from build123d import *

# Parameters (mm, degrees)
SKETCH037_W      = 2
SKETCH037_H      = 37
EXTRUDE036_DEPTH = 1
FILLET012_R      = 0.25
SKETCH038_W      = 13.25
SKETCH038_H      = 36
EXTRUDE037_DEPTH = 2
SKETCH031_W      = 37
SKETCH031_H      = 2.5
EXTRUDE029_DEPTH = 120
SKETCH030_W      = 56
SKETCH030_H      = 13.5
EXTRUDE028_DEPTH = 41
SKETCH036_W      = 120
SKETCH036_H      = 8
EXTRUDE035_DEPTH = 2
FILLET011_R      = 1
FILLET013_R      = 4
FILLET014_R      = 1


with BuildPart() as velcrobands:
    # Sketch037 → Extrude036 (new body)
    with BuildSketch(Plane.XY.offset(5.5)):
        with Locations((174, 26.5)):
            Rectangle(SKETCH037_W, SKETCH037_H)
        with Locations((147, 26.5)):
            Rectangle(SKETCH037_W, SKETCH037_H)
    extrude(amount=EXTRUDE036_DEPTH)

    # Fillet012
    fillet012_edges = [velcrobands.edges().sort_by_distance(p)[0] for p in [
        (148, 26.5, 6.5),
        (146, 26.5, 6.5),
        (173, 26.5, 6.5),
        (175, 26.5, 6.5),
    ]]
    fillet(fillet012_edges, radius=FILLET012_R)


with BuildPart() as sensorcuts:
    # Sketch038 → Extrude037 (new body)
    with BuildSketch(Plane.XY.offset(-0.75)):
        with Locations((151.375, 26.5)):
            Rectangle(SKETCH038_W, SKETCH038_H)
    extrude(amount=-EXTRUDE037_DEPTH)


with BuildPart() as extrude029:
    # Sketch031 → Extrude029 (new body)
    with BuildSketch(Plane.YZ.offset(56)):
        with Locations((26.412533, 0.5)):
            Rectangle(SKETCH031_W, SKETCH031_H)
    extrude(amount=EXTRUDE029_DEPTH)


with BuildPart() as band002:
    # Sketch030 → Extrude028 (new body)
    with BuildSketch(Plane.XZ.offset(-6)):
        Polygon((175, 5.5), (60, 5.5), (60, 17.5), (-4, 17.5), (-4, 2.5), (-122, 2.5), (-122, -2.5), (175, -2.5), align=None)
        with Locations((28, 6.75)):
            Rectangle(SKETCH030_W, SKETCH030_H, mode=Mode.SUBTRACT)
    extrude(amount=-EXTRUDE028_DEPTH)

    # Cut002: cut Extrude029
    add(extrude029.part, mode=Mode.SUBTRACT)

    # Cut005: cut sensorCuts
    add(sensorcuts.part, mode=Mode.SUBTRACT)


with BuildPart() as fillet014:
    # Sketch036 → Extrude035 (new body)
    with BuildSketch(Plane.XY.offset(2.5)):
        with Locations((-62, 43)):
            Rectangle(SKETCH036_W, SKETCH036_H)
        with Locations((-62, 10)):
            Rectangle(SKETCH036_W, SKETCH036_H)
    extrude(amount=EXTRUDE035_DEPTH)

    # Fillet011
    fillet011_edges = [fillet014.edges().sort_by_distance(p)[0] for p in [
        (-62, 14, 4.5),
        (-62, 6, 4.5),
        (-62, 47, 4.5),
        (-62, 39, 4.5),
    ]]
    fillet(fillet011_edges, radius=FILLET011_R)

    # Fusion011: union velcroBands, band002
    add(velcrobands.part)
    add(band002.part)

    # Fillet013
    fillet013_edges = [fillet014.edges().sort_by_distance(p)[0] for p in [
        (60, 26.5, 5.5),
        (60, 26.5, 17.5),
        (-4, 26.5, 17.5),
        (0, 26.5, 0),
        (0, 26.5, 13.5),
        (56, 26.5, 13.5),
    ]]
    fillet(fillet013_edges, radius=FILLET013_R)

    # Fillet014
    fillet014_edges = [fillet014.edges().sort_by_distance(p)[0] for p in [
        (119.5, 6, 5.5),
        (26.5, 6, -2.5),
        (28, 6, 17.5),
        (28, 6, 13.5),
        (119.5, 47, 5.5),
        (26.5, 47, -2.5),
        (158, 26.5, -2.5),
        (151.375, 8.5, -2.5),
        (144.75, 26.5, -2.5),
        (151.375, 44.5, -2.5),
        (28, 47, 17.5),
        (56, 6.956266, 0),
        (56, 45.956266, 0),
        (28, 47, 13.5),
        (56, 26.412533, 1.75),
        (158, 8.5, -1.625),
        (158, 44.5, -1.625),
        (144.75, 8.5, -1.625),
        (144.75, 44.5, -1.625),
    ]]
    fillet(fillet014_edges, radius=FILLET014_R)


solid = fillet014.part
Geometry: final body of the model. Coordinates: model frame, mm. A direction names the side the tool comes from. Give positions to 0.01 mm unless a question says otherwise; leave off trailing zeros. Order: outer loops, then holes, each group sorted by start corner. A loop starts at its lowest first (then second) coordinate and runs counter-clockwise, first axis right, second up. Notation, with made-up numbers: (79, -20) - (136, -20) arc R19 cw to (136, 10) - close; hole circle Ø10 at (-1, -8.75). An arc over 180 degrees is marked (long way). Use CSV: the item, a comma, the result in double quotes.
1. Access query for faces 1 (the face through (115, 26, -0.75)), 2 (the face through (-64, 43, 4.5)), 3 (the face through (28, 26, 13.5)). Directions: +Z, -Z, +X, -X, +Y, -Y. A direction counts if a zero-diameter tool reaches every point of the face in a straight line with its end or side. Return the directions, or none.
Answers below:
face 1,"+X"
face 2,"+Z, -X, +Y, -Y"
face 3,"+Y, -Y"
2. Section query A-A (x = 19.5). Output: boundary loops of the cut face in (y, z).
Answers below:
outline,"(6, -1.5) arc R1 ccw to (7, -2.5) - (46, -2.5) arc R1 ccw to (47, -1.5) - (47, -1) arc R1 ccw to (46, 0) - (7, 0) arc R1 ccw to (6, -1) - close; (6, 14.5) arc R1 ccw to (7, 13.5) - (46, 13.5) arc R1 ccw to (47, 14.5) - (47, 16.5) arc R1 ccw to (46, 17.5) - (7, 17.5) arc R1 ccw to (6, 16.5) - close"
3. Mould query, pull axis Y, two halves, no side actions, for faces 4 (the face through (115, 26, 1.75)), 5 (the face through (37, 6, 16)), 6 (the face through (175, 26, 2)), 7 (the face through (-62, 26, 2.5)). Classes: +Y half, -Y half, draft (parallel to the pull), parting line (faces both ways), or undercut.
Answers below:
face 4,"undercut"
face 5,"-Y half"
face 6,"draft"
face 7,"undercut"
4. Contact query for flat-ended pins moving along their axis: pin 1 (0.6 mm diameter, centred on y = 27, z = 6, fed in from -X); pin 2 (12 mm diameter, centred on x = 133, y = 15.5, fed in from +Z); pin 3 (3 mm diameter, centred on x = -50, y = 42.5, fed in from +Z). Output: stop coordinate, or through.
Answers below:
pin 1,"x = -4"
pin 2,"z = 5.5"
pin 3,"z = 4.5"
5. Section query C-C (x = 70). Output: boundary loops of the cut face in (y, z).
Answers below:
outline,"(6, -1.5) arc R1 ccw to (7, -2.5) - (46, -2.5) arc R1 ccw to (47, -1.5) - (47, 4.5) arc R1 ccw to (46, 5.5) - (7, 5.5) arc R1 ccw to (6, 4.5) - close; hole (7.91, -0.75) - (44.91, -0.75) - (44.91, 1.75) - (7.91, 1.75) - close"
6. Material intervals for line 1 along Z through (x, y) = (18, 37); line 2 along Z through (x, y) = (90.5, 11.5); line 3 along X through (y, z) = (38.5, 9.5), sorted ascending. Write a range as from..to.
Answers below:
line 1,"-2.5..0, 13.5..17.5"
line 2,"-2.5..-0.75, 1.75..5.5"
line 3,"-4..0, 56..60"
7. Section query B-B (x = -69). Output: boundary loops of the cut face in (y, z), plus the area to 3 significant figures.
Answers below:
outline,"(6, -1.5) arc R1 ccw to (7, -2.5) - (46, -2.5) arc R1 ccw to (47, -1.5) - (47, 3.5) arc R1 ccw to (46, 4.5) - (40, 4.5) arc R1 ccw to (39, 3.5) - (39, 2.5) - (14, 2.5) - (14, 3.5) arc R1 ccw to (13, 4.5) - (7, 4.5) arc R1 ccw to (6, 3.5) - close"
area,"236 mm2"
